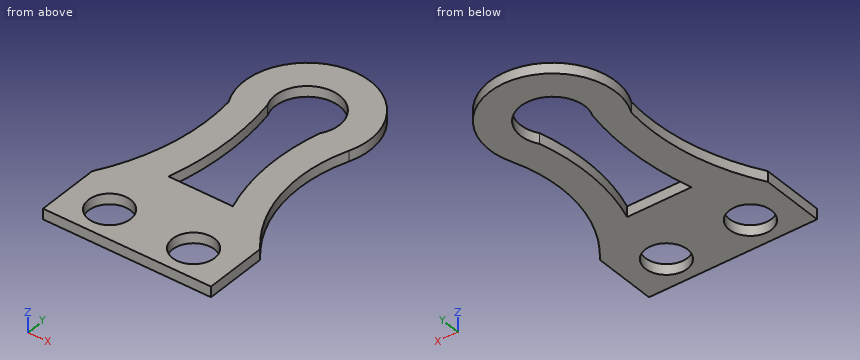
Autodesk Inventor part; units mm, degrees
ref_plane "YZ Plane" through (0, 0, 0) normal (1, 0, 0) x (0, 1, 0)
ref_plane "XZ Plane" through (0, 0, 0) normal (0, 1, 0) x (-1, 0, 0)
ref_plane "XY Plane" through (0, 0, 0) normal (0, 0, 1) x (1, 0, 0)
sketch "Sketch1" plane through (0, 0, 0) normal (0, 0, 1) x (1, 0, 0)
  arc A0 (35.3023, -14.3304) -> (-33.6082, -17.9471) centre (0, 0) ccw
  circle A1 centre (0, 0) radius 19.431
  arc A2 (19.431, 0) -> (19.431, -82.55) centre (138.6611, -41.275) ccw
  arc A3 (-19.431, -82.55) -> (-19.431, 0) centre (-184.2713, -41.275) ccw
  line L0 (-19.431, -82.55) -> (19.431, -82.55)
  arc A4 (35.6836, -13.3526) -> (57.2802, -108.5447) centre (118.9453, -44.5086) ccw
  line L1 (0, -139.7) -> (50.8, -139.7)
  line L2 (50.8, -139.7) -> (50.8, -101.6)
  line L3 (-50.8, -101.6) -> (-50.8, -139.7)
  line L4 (-50.8, -139.7) -> (0, -139.7)
  arc A5 (-50.8, -101.6) -> (-33.6082, -17.9471) centre (-161.9278, -35.1687) ccw
  line L5 (-50.8, -139.7) -> (-25.4, -139.7)
  circle A6 centre (-25.4, -120.65) radius 12.7
  line L6 (50.8, -139.7) -> (25.4, -139.7)
  circle A7 centre (25.4, -120.65) radius 12.7
  dimension "d0" = 76.2
  dimension "d1" = 38.862
  dimension "d5" = 177.8
  dimension "d12" = 101.6
  dimension "d13" = 38.1
  dimension "d14" = 139.7
  dimension "d20" = 25.4
  dimension "d21" = 25.4
  dimension "d23" = 25.4
extrude "Extrusion1" add sketch "Sketch1" along normal blind 6.35
properties part number "4-4"
Could you check a few things on this model? Use its own coordinates, in mm. Give positions to 0.01 mm unless a question says otherwise; leave off trailing zeros. Order: outer loops, then holes, each group sorted by start corner. A loop starts at its lowest first (then second) coordinate and runs counter-clockwise, first axis right, second up. Notation, with made-up numbers: (-5, 39.5) - (35, 39.5) arc R20 cw to (35, 53.5) - close; hole circle Ø10 at (26, 47.25). An arc over 180 degrees is marked (long way). One line per question, with ' | ' between items. Start each with the question number.
Item 1: I want a section at B-B on x = 0. Write out the boundary of the cut face in (y, z).
Item 2: I need wall thicknesses on probe 1 along Y at (x, z) = (0, 5); probe 2 along X at (y, z) = (0, 3.25); probe 3 along X at (y, z) = (-125.5, 2.75). Which ranges of each line are inside material? Lowest first, please. Write a range as [from, to].
Item 3: I'm going to push flat-ended pins straight in: pin 1 Ø1.5 at (y, z) = (-12.5, 5.5) entering from -X; pin 2 Ø3 at (y, z) = (-33.5, 1) entering from -X; pin 3 Ø3 at (x, z) = (-3, 2.5) entering from +Y; pin 4 Ø1 at (x, y) = (14, -69) entering from +Z. Where does each tip first touch, or does it pass through?
Item 4: I want a section at D-D on x = -35.5. Write out the boundary of the cut face in (y, z), then the cut area to 3 significant figures.
Item 5: I want a section at C-C on y = -110.5. Write out the boundary of the cut face in (x, z).
Item 6: I want a section at A-A on y = 0. Write out the boundary of the cut face in (x, z).
Verdict:
1) outline: (-139.7, 0) - (-82.55, 0) - (-82.55, 6.35) - (-139.7, 6.35) - close; (19.43, 0) - (38.1, 0) - (38.1, 6.35) - (19.43, 6.35) - close
2) probe 1: [-139.7, -82.55], [19.43, 38.1] | probe 2: [-38.1, -19.43], [19.43, 38.1] | probe 3: [-50.8, -37.14], [-13.66, 13.66], [37.14, 50.8]
3) pin 1: x = -36.24 | pin 2: x = -32.5 | pin 3: y = 38.07 | pin 4: through
4) outline: (-139.7, 0) - (-128.35, 0) - (-128.35, 6.35) - (-139.7, 6.35) - close; (-112.95, 0) - (-63.07, 0) - (-63.07, 6.35) - (-112.95, 6.35) - close; (-13.83, 0) - (13.83, 0) - (13.83, 6.35) - (-13.83, 6.35) - close | area: 564 mm^2
5) outline: (-50.8, 0) - (-33.03, 0) - (-33.03, 6.35) - (-50.8, 6.35) - close; (-17.77, 0) - (17.77, 0) - (17.77, 6.35) - (-17.77, 6.35) - close; (33.03, 0) - (50.8, 0) - (50.8, 6.35) - (33.03, 6.35) - close
6) outline: (-38.1, 0) - (-19.43, 0) - (-19.43, 6.35) - (-38.1, 6.35) - close; (19.43, 0) - (38.1, 0) - (38.1, 6.35) - (19.43, 6.35) - close
